```python
from build123d import *

# Parameters (mm, degrees)
PAD_DEPTH       = 8
POCKET_DEPTH    = 5.001
SKETCH002_R     = 4
POCKET001_DEPTH = 12
CHAMFER_SIZE    = 4
CHAMFER001_SIZE = 1
CHAMFER002_SIZE = 1


with BuildPart() as part:
    # Sketch → Pad (new body, symmetric)
    with BuildSketch(Plane.XZ):
        with BuildLine():
            Line((-22, -15), (22, -15))
            Line((22, -15), (22, -10))
            Line((22, -10), (7, -10))
            Line((7, -10), (7, 0))
            ThreePointArc((7, 0), (0, 7), (-7, 0))
            Line((-7, -10), (-7, 0))
            Line((-22, -10), (-7, -10))
            Line((-22, -15), (-22, -10))
        make_face()
    extrude(amount=PAD_DEPTH, both=True)

    # Sketch001 (on Face7 of Pad) → Pocket (cut, through all)
    with BuildSketch(Plane(origin=(0, 0, -10), x_dir=(-1, 0, 0), z_dir=(0, 0, 1))):
        with BuildLine():
            ThreePointArc((-15, 2.5), (-17.5, 0), (-15, -2.5))
            Line((-15, -2.5), (-12, -2.5))
            ThreePointArc((-12, -2.5), (-9.5, 0), (-12, 2.5))
            Line((-15, 2.5), (-12, 2.5))
        make_face()
        with BuildLine():
            ThreePointArc((12, 2.5), (9.5, 0), (12, -2.5))
            Line((12, -2.5), (15, -2.5))
            ThreePointArc((15, -2.5), (17.5, 0), (15, 2.5))
            Line((12, 2.5), (15, 2.5))
        make_face()
    extrude(amount=-POCKET_DEPTH, mode=Mode.SUBTRACT)

    # Sketch002 (on Face3 of Pocket) → Pocket001 (cut)
    with BuildSketch(Plane(origin=(0, 8, 0), x_dir=(1, 0, 0), z_dir=(0, 1, 0))):
        Circle(SKETCH002_R)
    extrude(amount=-POCKET001_DEPTH, mode=Mode.SUBTRACT)

    # Chamfer
    chamfer_edges = [part.edges().sort_by_distance(p)[0] for p in [
        (22, 8, -12.5),
        (-22, 8, -12.5),
        (-22, -8, -12.5),
        (22, -8, -12.5),
    ]]
    chamfer(chamfer_edges, length=CHAMFER_SIZE)

    # Chamfer001
    chamfer001_edges = [part.edges().sort_by_distance(p)[0] for p in [
        (-12.5, 8, -10),
        (-20, 6, -10),
        (-22, 0, -10),
        (-12.5, -8, -10),
        (12.5, -8, -10),
        (20, -6, -10),
        (22, 0, -10),
        (20, 6, -10),
        (12.5, 8, -10),
        (-20, -6, -10),
        (0, -8, 7),
    ]]
    chamfer(chamfer001_edges, length=CHAMFER001_SIZE)

    # Chamfer002
    chamfer002_edges = [part.edges().sort_by_distance(p)[0] for p in [
        (-4, 8, 0),
    ]]
    chamfer(chamfer002_edges, length=CHAMFER002_SIZE)


solid = part.part
```
For this review, take the finished solid that the model builds, in its own axes (mm). A direction names the side the tool comes from. Coordinates: 2 decimals unless noted, no trailing zeros. Write each loop counter-clockwise with the first axis right and the second up, starting at its lowest first coordinate (ties: lowest second). Pieces come first, ordered by that corner, then holes. Notation, with made-up numbers: (-27, -6.5) - (-15, -6.5) arc R25 cw to (-15, 10.5) - close; hole circle Ø10 at (-3.5, 72.5). An arc over 180 degrees is marked (long way). Answer in a Markdown table with one row per item. Add a question column.
Q1. We need section C-C, the plane z = -6.5. State the section outline as (x, y) points, and give its area (3 significant figures).
Q2. We need section A-A, the plane y = 0. State the section outline as (x, z) points, and give its area (3 significant figures).
Q3. For P1, Ø5.5, axis at y = 1.5, z = -5, coming from the -X side; P2, Ø5.5, axis at y = 2.5, z = -5, coming from the +X side; P3, Ø2, axis at x = -2.5, y = -2.5, coming from the +Z side, all flat-tipped, find the tip position at first contact; note any pin that passes through.
Q4. We need section B-B, the plane y = -3. State the section outline as (x, z) points, and give its area (3 significant figures).
Q5. Draft analysis for pull direction Y (two halves, no side actions). For faces 6 (the flat face through (-6.5, -7.5, -5.4)), 7 (the flat face through (14, 2.5, -12)), 8 (the flat face through (19.61, 5.67, -10.49)), state which applies: +Y half, -Y half, draft (parallel to the pull), parting line (faces both ways), or undercut.
Q6. Tool access review of faces 1 (the flat face through (6.5, -7.5, -5.6)), 2 (the cylindrical face through (-9.5, -0.1, -12.5)), 3 (the flat face through (-21.5, -0.1, -10.5)), 4 (the flat face through (-12.1, -7.5, -10.5)), 5 (the cylindrical face through (-0.867, 1.577, 3.905)): name each direction out of +Z, -Z, +X, -X, +Y, -Y from which nothing blocks a thin tool from reaching the whole face with its end or side.
Q7. For probe 1 along X at (y, z) = (2, 0); probe 2 along Z at (x, y) = (0, 1.5); probe 3 along Z at (x, y) = (15, -7), list the stretches that pass through material, from the lowest coordinate up.
Q8. We need section D-D, the plane x = 18.5. State the section outline as (y, z) points.
Answer list:
| question | item | result |
|---|---|---|
| 1 | outline | (-7, -7) - (-6, -8) - (6, -8) - (7, -7) - (7, 8) - (-7, 8) - close |
| 1 | area | 223 mm2 |
| 2 | outline | (-22, -15) - (-17.5, -15) - (-17.5, -10) - (-21, -10) - (-22, -11) - close; (-9.5, -15) - (9.5, -15) - (9.5, -10) - (7, -10) - (7, 0) arc R7 ccw to (-7, 0) - (-7, -10) - (-9.5, -10) - close; (17.5, -15) - (22, -15) - (22, -11) - (21, -10) - (17.5, -10) - close; hole circle Ø8 at (0, 0) |
| 2 | area | 306 mm2 |
| 3 | P1 | stops at x = -7 |
| 3 | P2 | stops at x = 7 |
| 3 | P3 | stops at z = 6.84 |
| 4 | outline | (-22, -15) - (22, -15) - (22, -11) - (21, -10) - (7, -10) - (7, 0) arc R7 ccw to (-7, 0) - (-7, -10) - (-21, -10) - (-22, -11) - close; hole circle Ø8 at (0, 0) |
| 4 | area | 386 mm2 |
| 5 | face 6 | -Y half |
| 5 | face 7 | undercut |
| 5 | face 8 | +Y half |
| 6 | face 1 | +Z, +X, -Y |
| 6 | face 2 | +Z, -Z |
| 6 | face 3 | +Z, -X, +Y, -Y |
| 6 | face 4 | +Z, -X, -Y |
| 6 | face 5 | +Y |
| 7 | probe 1 | x = -7 to -4, 4 to 7 |
| 7 | probe 2 | z = -15 to -4, 4 to 7 |
| 7 | probe 3 | z = -15 to -10 |
| 8 | outline | (-7.5, -15) - (7.5, -15) - (7.5, -11) - (6.09, -10) - (-6.09, -10) - (-7.5, -11) - close |
